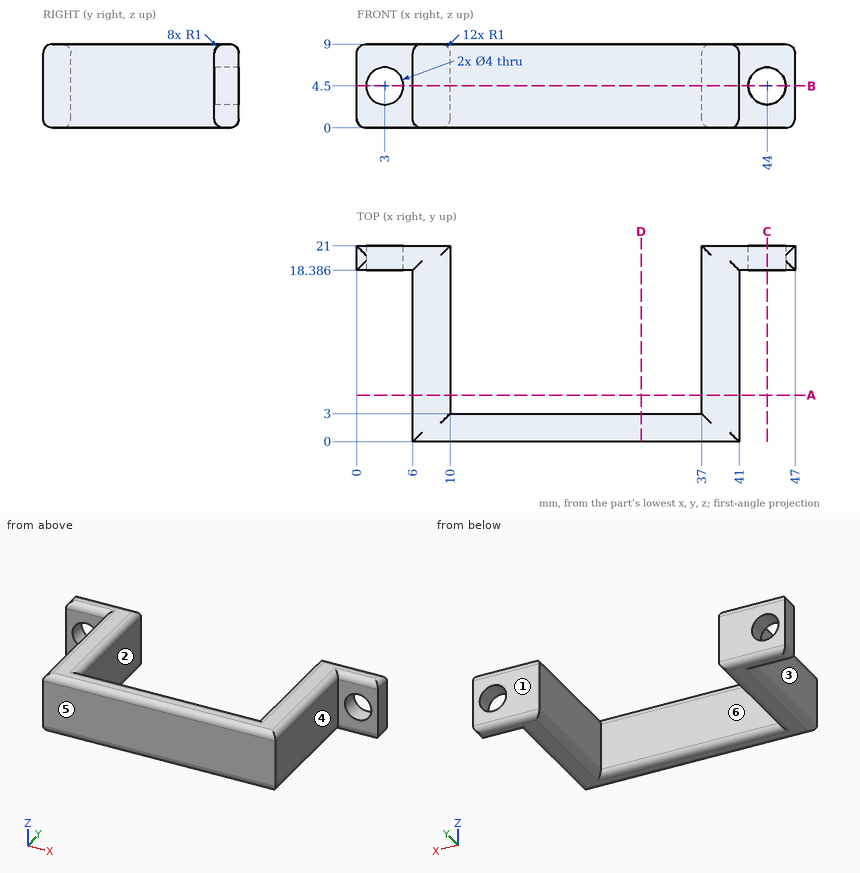
Can you work these out from the drawing? Everything is in mm from the part's minimum corner. A direction names the side the tool comes from. Coordinates: 2 decimals unless noted, no trailing zeros. Loops run counter-clockwise (first coordinate to the right, second up) from the corner with the lowest first, then second, coordinate; pieces in that order, holes last. Notation, with made-up numbers: (6.5, 77) -> (23.5, 77) arc R31 cw to (23.5, 106) -> close; hole circle Ø8 at (-3, 19.5). An arc over 180 degrees is marked (long way). Return JSON: item names as keys, results as strings.
1) If we section it at A-A, the plane y = 5: Write out the boundary of the cut face in (x, z).
Results below:
{"outline": "(6, 1) arc R1 ccw to (7, 0) -> (9, 0) arc R1 ccw to (10, 1) -> (10, 8) arc R1 ccw to (9, 9) -> (7, 9) arc R1 ccw to (6, 8) -> close; (37, 1) arc R1 ccw to (38, 0) -> (40, 0) arc R1 ccw to (41, 1) -> (41, 8) arc R1 ccw to (40, 9) -> (38, 9) arc R1 ccw to (37, 8) -> close"}
2) For the marked faces 1, 2 and 3, which set-ups out of +Z, -Z, +X, -X, +Y, -Y let a thin tool reach every point of the face, with its end or its side?
Results below:
{"face 1": "+Z, -Z, +X, -X, +Y", "face 2": "+Z, -Z, +Y", "face 3": "+Z, -Z, -X, -Y"}
3) I need wall thicknesses on line 1 (X direction, y = 14.25, z = 6.5); line 2 (Z direction, x = 3, y = 19.95); line 3 (Y direction, x = 15, z = 4). Which ranges of each line are inside material? Lowest first, please. Write a range as from..to.
Results below:
{"line 1": "6..10, 37..41", "line 2": "0..2.5, 6.5..9", "line 3": "0..3"}
4) If we section it at B-B, the plane z = 4.5: Write out the boundary of the cut face in (x, y) (1 decimal).
Results below:
{"outline": "(0, 18.4) -> (1, 18.4) -> (1, 21) -> (0, 21) -> close; (5, 18.4) -> (6, 18.4) -> (6, 0) -> (41, 0) -> (41, 18.4) -> (42, 18.4) -> (42, 21) -> (37, 21) -> (37, 3) -> (10, 3) -> (10, 21) -> (5, 21) -> close; (46, 18.4) -> (47, 18.4) -> (47, 21) -> (46, 21) -> close"}
5) Thinking about a two-plate mould opening in X: for the marked faces 4, 5 and 6, which applies, +X half, -X half, draft (parallel to the pull), parting line (faces both ways), or undercut?
Results below:
{"face 4": "+X half", "face 5": "draft", "face 6": "undercut"}
6) Will these pins go through, and if not, where does the flat tip stop? pin 1 (2.5 mm diameter, centred on x = 44, z = 4.5, fed in from -Y); pin 2 (2 mm diameter, centred on y = 6, z = 3.5, fed in from -X); pin 3 (5 mm diameter, centred on y = 15, z = 6.5, fed in from +X).
Results below:
{"pin 1": "through", "pin 2": "x = 6", "pin 3": "x = 41"}
7) If we section it at D-D, the plane x = 30.5: Write out the boundary of the cut face in (y, z).
Results below:
{"outline": "(0, 1) arc R1 ccw to (1, 0) -> (2, 0) arc R1 ccw to (3, 1) -> (3, 8) arc R1 ccw to (2, 9) -> (1, 9) arc R1 ccw to (0, 8) -> close"}
8) If we section it at C-C, the plane x = 44: Write out the boundary of the cut face in (y, z) (1 decimal), then the cut area to 3 significant figures.
Results below:
{"outline": "(18.4, 1) arc R1 ccw to (19.4, 0) -> (20, 0) arc R1 ccw to (21, 1) -> (21, 2.5) -> (18.4, 2.5) -> close; (18.4, 6.5) -> (21, 6.5) -> (21, 8) arc R1 ccw to (20, 9) -> (19.4, 9) arc R1 ccw to (18.4, 8) -> close", "area": "12.2 mm²"}
